Here's how the part is built. I have some questions about the finished solid (model axes, mm). A direction names the side the tool comes from. Give positions to 0.01 mm unless a question says otherwise; leave off trailing zeros. Order: outer loops, then holes, each group sorted by start corner. A loop starts at its lowest first (then second) coordinate and runs counter-clockwise, first axis right, second up. Notation, with made-up numbers: M -31,57.5 L 6,57.5 A6 ccw 6,66.5 Z; hole C 87.5,-28 d10. An arc over 180 degrees is marked long. Use one line per item in the form item = value.
from build123d import *

# Parameters (mm, degrees)
BOSS_EXTRUDE1_DEPTH = 4
SKETCH2_R           = 2
SKETCH2_R_2         = 1.5
CUT_EXTRUDE1_DEPTH  = 95.026591983
SKETCH4_W           = 20
SKETCH4_H           = 100
BOSS_EXTRUDE2_DEPTH = 4
FILLET3_R           = 42
FILLET4_R           = 12
SKETCH7_R           = 2
CUT_EXTRUDE3_DEPTH  = 105.120122935
CHAMFER1_SIZE       = 10
FILLET8_R           = 2
CUT_EXTRUDE4_DEPTH  = 105.120122935
CUT_EXTRUDE5_DEPTH  = 105.120122935
SKETCH10_R          = 2
CUT_EXTRUDE6_DEPTH  = 105.120122935


with BuildPart() as part:
    # Sketch1 → Boss-Extrude1 (new body)
    with BuildSketch(Plane.XY):
        Polygon((-40, 60), (-25, 60), (-25, 52), (-15, 52), (-15, 0), (-21, 0), (-21, -50), (21, -50), (21, 0), (15, 0), (15, 52), (25, 52), (25, 60), (40, 60), (40, -60), (22, -60), (22, -85), (12, -85), (12, -60), (-12, -60), (-12, -85), (-22, -85), (-22, -60), (-40, -60), align=None)
    extrude(amount=BOSS_EXTRUDE1_DEPTH)

    # Sketch2 → Cut-Extrude1 (cut, through all)
    with BuildSketch(Plane(origin=(0, 0, 0), x_dir=(-1, 0, 0), z_dir=(0, 0, -1))):
        with Locations((-28.5, -32)):
            Circle(SKETCH2_R)
        with Locations((17, -56.5)):
            Circle(SKETCH2_R_2)
        with Locations((28.8, -32)):
            Circle(SKETCH2_R)
        with Locations((-17, -56.5)):
            Circle(SKETCH2_R_2)
    extrude(amount=-CUT_EXTRUDE1_DEPTH, mode=Mode.SUBTRACT)

    # Sketch4 → Boss-Extrude2 (add)
    with BuildSketch(Plane.XY.offset(4)):
        with Locations((-50, 10)):
            Rectangle(SKETCH4_W, SKETCH4_H)
        with Locations((50, 10)):
            Rectangle(SKETCH4_W, SKETCH4_H)
    extrude(amount=-BOSS_EXTRUDE2_DEPTH)

    # Fillet3
    # the kernel refuses this fillet: 42 mm, written as the material it takes off along each edge
    with BuildSketch(Plane(origin=(60, 60, 107.531396204), x_dir=(0, -1, 0), z_dir=(0, 0, -1))) as fillet3_piece_1:
        with BuildLine():
            CenterArc((41.412558482, 42), FILLET3_R, 189.594068227, 80.405931773)
            Line((0, 35), (-0.82825117, 34.86))
            ThreePointArc((-0.82825117, 34.86), (-0.84, 17.5), (-0.84, 0))
            Line((-0.84, 0), (0, -0.84))
            Line((0, -0.84), (41.412558482, -0.84))
            Line((41.412558482, -0.84), (41.412558482, 0))
        make_face()
    extrude(amount=211.062792409, mode=Mode.SUBTRACT)
    with BuildSketch(Plane(origin=(-60, 60, 107.531396204), x_dir=(1, 0, 0), z_dir=(0, 0, -1))) as fillet3_piece_2:
        with BuildLine():
            CenterArc((42, 41.412558482), FILLET3_R, 180, 80.405931773)
            Line((0, 41.412558482), (-0.84, 41.412558482))
            Line((-0.84, 41.412558482), (-0.84, 0))
            Line((-0.84, 0), (0, -0.84))
            ThreePointArc((0, -0.84), (17.5, -0.84), (34.86, -0.82825117))
            Line((34.86, -0.82825117), (35, 0))
        make_face()
    extrude(amount=211.062792409, mode=Mode.SUBTRACT)

    # Fillet4
    fillet4_edges = [part.edges().sort_by_distance(p)[0] for p in [
        (60, -40, 2),
        (-60, -40, 2),
    ]]
    fillet(fillet4_edges, radius=FILLET4_R)

    # Sketch7 → Cut-Extrude3 (cut, through all)
    with BuildSketch(Plane.XY):
        with Locations(Location((-55, -20, 0), (0, 0, 180))):
            Circle(SKETCH7_R)
        with Locations(Location((55, -20, 0), (0, 0, 180))):
            Circle(SKETCH7_R)
        with Locations(Location((-37, -20, 0), (0, 0, 180))):
            Circle(SKETCH7_R)
        with Locations(Location((37, -20, 0), (0, 0, 180))):
            Circle(SKETCH7_R)
    extrude(amount=CUT_EXTRUDE3_DEPTH, mode=Mode.SUBTRACT)

    # Chamfer1
    chamfer1_edges = [part.edges().sort_by_distance(p)[0] for p in [
        (-40, -60, 2),
        (40, -60, 2),
    ]]
    chamfer(chamfer1_edges, length=CHAMFER1_SIZE)

    # Fillet8
    fillet8_edges = [part.edges().sort_by_distance(p)[0] for p in [
        (-30, -60, 2),
        (-40, -50, 2),
        (30, -60, 2),
        (40, -50, 2),
        (40, -40, 2),
        (-40, -40, 2),
    ]]
    fillet(fillet8_edges, radius=FILLET8_R)

    # Sketch8 → Cut-Extrude4 (cut, through all)
    with BuildSketch(Plane(origin=(0, 0, 0), x_dir=(-1, 0, 0), z_dir=(0, 0, -1))):
        with BuildLine():
            ThreePointArc((-17.964817996, 17.438774634), (-30.770630407, 21.535466224), (-44.214817996, 21.375674028))
            ThreePointArc((-44.214817996, 21.375674028), (-45.841525426, 19.061841075), (-43.527692473, 17.435133644))
            ThreePointArc((-43.527692473, 17.435133644), (-31.363903701, 17.579707536), (-19.777692473, 13.87317705))
            ThreePointArc((-19.777692473, 13.87317705), (-17.088456442, 14.749538603), (-17.964817996, 17.438774634))
        make_face()
        with BuildLine():
            ThreePointArc((17.964817996, 17.438774634), (30.770630407, 21.535466224), (44.214817996, 21.375674028))
            ThreePointArc((44.214817996, 21.375674028), (45.841525426, 19.061841075), (43.527692473, 17.435133644))
            ThreePointArc((43.527692473, 17.435133644), (31.363903701, 17.579707536), (19.777692473, 13.87317705))
            ThreePointArc((19.777692473, 13.87317705), (17.088456442, 14.749538603), (17.964817996, 17.438774634))
        make_face()
    extrude(amount=-CUT_EXTRUDE4_DEPTH, mode=Mode.SUBTRACT)

    # Sketch9 → Cut-Extrude5 (cut, through all)
    with BuildSketch(Plane.XY.offset(4)):
        Polygon((-24, 52), (-20, 52), (-20, 45.2), (-18.25, 45.2), (-18.25, 42), (-25.75, 42), (-25.75, 45.2), (-24, 45.2), align=None)
    cut_extrude5 = extrude(amount=-CUT_EXTRUDE5_DEPTH, mode=Mode.SUBTRACT)

    # Mirror1: Cut-Extrude5 across plane
    add(cut_extrude5.mirror(Plane(origin=(0, 0, 0), x_dir=(0, 0, 1), z_dir=(1, 0, 0))), mode=Mode.SUBTRACT)

    # Sketch10 → Cut-Extrude6 (cut, through all)
    with BuildSketch(Plane.XY.offset(4)):
        with Locations(Location((55, -20, 0), (0, 0, 180))):
            Circle(SKETCH10_R)
        with BuildLine():
            Line((55, -5), (60, -5))
            Line((60, -5), (60, -15))
            Line((60, -15), (55, -15))
            ThreePointArc((55, -15), (52.886908691, -15.468461065), (51.169777784, -16.786061952))
            ThreePointArc((51.169777784, -16.786061952), (44.12561752, -17.402346119), (43.509333353, -10.358185855))
            ThreePointArc((43.509333353, -10.358185855), (48.660726074, -6.405383194), (55, -5))
        make_face()
    cut_extrude6 = extrude(amount=-CUT_EXTRUDE6_DEPTH, mode=Mode.SUBTRACT)

    # Mirror2: Cut-Extrude6 across plane
    add(cut_extrude6.mirror(Plane(origin=(0, 0, 0), x_dir=(0, 0, 1), z_dir=(1, 0, 0))), mode=Mode.SUBTRACT)


solid = part.part
Q1. I want a section at D-D on z = 0.75. State how many separate pieces and enclosed holes the cut face has, then the cut area to 3 significant figures.
Found:
separate_pieces = 1
enclosed_holes = 10
area = 8,390 mm²
Q2. On a 3-axis mill with a long thin cutter (end or side, diameter ignored), from which of +Z, -Z, +X, -X, +Y, -Y can I reach the whole of each face in a straight line? I mean faces 5 (the face through (-60, 7, 2)), 6 (the face through (31.5, 17.6, 2)), 7 (the face through (45, -40, 2)), 8 (the face through (26, -11, 0)), 9 (the face through (-20, 49, 2)). Say none if no direction works.
Found:
face_5 = +Z, -Z, -X, +Y, -Y
face_6 = +Z, -Z
face_7 = +Z, -Z, +X, -Y
face_8 = -Z, +X, -X, +Y, -Y
face_9 = +Z, -Z, +Y
Q3. Thinking about a two-plate mould opening in X: for faces 1 (the face through (-22, -73, 2)), 2 (the face through (60, -22, 2)), 3 (the face through (26, -60, 2)), 4 (the face through (17, 52, 2)), which applies, +X half, -X half, draft (parallel to the pull), parting line (faces both ways), or undercut?
Found:
face_1 = -X half
face_2 = +X half
face_3 = draft
face_4 = undercut
Q4. I want a section at A-A on y = -45. Write out the boundary of the cut face in (x, z), then the cut area to 3 significant figures.
Found:
outline = M -40,0 L -21,0 L -21,4 L -40,4 Z; M 21,0 L 40,0 L 40,4 L 21,4 Z
area = 152 mm²
Q5. I need wall thicknesses on L1, parallel to Y at x = -28.8, z = 3.05; L2, parallel to X at y = 6, z = 3.55; L3, parallel to X at y = 45.5, z = 0.45. Which ranges of each line are inside material? Lowest first, please.
Found:
L1 = -60 to -34, -30 to 17.1, 21.19 to 59.18
L2 = -60 to -15, 15 to 60
L3 = -50.24 to -24, -20 to -15, 15 to 20, 24 to 50.24
Q6. I want a section at B-B on x = -1. Write out the boundary of the cut face in (y, z).
Found:
outline = M -60,0 L -50,0 L -50,4 L -60,4 Z
Q7. I want a section at C-C on y = 37.5. Write out the boundary of the cut face in (x, z), then the cut area to 3 significant figures.
Found:
outline = M -55.5,0 L -15,0 L -15,4 L -55.5,4 Z; M 15,0 L 55.5,0 L 55.5,4 L 15,4 Z
area = 324 mm²
Q8. I'm going to push flat-ended pins straight in: pin 1 Ø1.4 at (x, z) = (25.5, 3) entering from -Y; pin 2 Ø0.8 at (x, z) = (-24.5, 1.5) entering from +Y; pin 3 Ø2 at (y, z) = (55, 1) entering from +X; pin 4 Ø3 at (x, y) = (-25, 13) entering from -Z. Where does each tip first touch, or does it pass through?
Found:
pin_1 = -60
pin_2 = 52
pin_3 = 40.58
pin_4 = 0
